from build123d import *

# Parameters (mm, degrees)
F0_W     = 152.4
F0_H     = 127
F1_DEPTH = 127
F2_W     = 101.6
F2_H     = 76.2
F3_DEPTH = 75.946
F4_R     = 23.2368410965
F5_DEPTH = 177.8
F6_R     = 38.1
F7_SIZE  = 35.56
F8_W     = 44.2467968255
F8_H     = 50.8
F9_DEPTH = 57.912


# Not quite as in the source:
# - a feature names something its author has since deleted; it is built from what else it names


with BuildPart() as f1:
    # F0 (on Front) → F1 (new body)
    with BuildSketch(Plane.XZ):
        Rectangle(F0_W, F0_H)
    extrude(amount=F1_DEPTH)

    # F2 (on face) → F3 (cut)
    with BuildSketch(Plane.XY.offset(63.5)):
        with Locations((25.4, -88.9)):
            Rectangle(F2_W, F2_H)
    extrude(amount=-F3_DEPTH, mode=Mode.SUBTRACT)

    # F4 (on face) → F5 (cut)
    with BuildSketch(Plane.XY.offset(-12.446)):
        with Locations((25.4, -88.9)):
            Circle(F4_R)
    extrude(amount=-F5_DEPTH, mode=Mode.SUBTRACT)

    # F6
    f6_edges = [f1.edges().sort_by_distance(p)[0] for p in [
        (-50.8, -127, 63.5),
    ]]
    fillet(f6_edges, radius=F6_R)

    # F7
    f7_edges = [f1.edges().sort_by_distance(p)[0] for p in [
        (76.2, -25.4, 63.5),
    ]]
    chamfer(f7_edges, length=F7_SIZE)

    # F8 (on face) → F9 (cut)
    with BuildSketch(Plane.XY.offset(63.5)):
        with Locations((-3.2766015872, -25.4)):
            Rectangle(F8_W, F8_H)
    extrude(amount=-F9_DEPTH, mode=Mode.SUBTRACT)


solid = f1.part
Design review of the part built by this model. Coordinates are the model's own, in mm. A direction names the side the tool comes from. Give positions to 0.01 mm unless a question says otherwise; leave off trailing zeros. Order: outer loops, then holes, each group sorted by start corner. A loop starts at its lowest first (then second) coordinate and runs counter-clockwise, first axis right, second up.
1. Add section A-A, the plane x = 25.4. State the section outline as (y, z) points.
Solution:
outline: (-127, -63.5) - (-112.14, -63.5) - (-112.14, -12.45) - (-127, -12.45) - close; (-65.66, -63.5) - (0, -63.5) - (0, 63.5) - (-50.8, 63.5) - (-50.8, -12.45) - (-65.66, -12.45) - close
2. Mouldability with a two-part tool opening along X and no side actions: class faces 1 (the flat face through (18.847, -26, 35)), 2 (the flat face through (58.67, -25.04, 45.47)), 3 (the flat face through (-51, -44, 63.5)) as +X half, -X half, draft (parallel to the pull), parting line (faces both ways), or undercut.
Solution:
face 1: undercut
face 2: +X half
face 3: draft
3. Add section B-B, the plane y = -30.5. State the section outline as (x, z) points.
Solution:
outline: (-76.2, -63.5) - (76.2, -63.5) - (76.2, 27.94) - (40.64, 63.5) - (18.85, 63.5) - (18.85, 5.59) - (-25.4, 5.59) - (-25.4, 63.5) - (-76.2, 63.5) - close
4. Add section C-C, the plane z = -36.5. State the section outline as (x, y) points.
Solution:
outline: (-76.2, -127) - (76.2, -127) - (76.2, 0) - (-76.2, 0) - close; hole circle Ø46.47 at (25.4, -88.9)
5. Add section D-D, the plane y = -97.5. State the section outline as (x, z) points, then the cut area to 3 significant figures.
Solution:
outline: (-76.2, -63.5) - (3.81, -63.5) - (3.81, -12.45) - (-25.4, -12.45) - (-25.4, 62.52) - (-76.2, 62.52) - close; (46.99, -63.5) - (76.2, -63.5) - (76.2, -12.45) - (46.99, -12.45) - close
area: 9,380 mm2
6. For pin 1 Ø5 at (x, y) = (58.5, -61) entering from +Z; pin 2 Ø6 at (x, z) = (20.5, -0.5) entering from +Y; pin 3 Ø5 at (y, z) = (-83, 49) entering from +X, all flat-tipped, find the tip position at first contact; note any pin that passes through.
Solution:
pin 1: stops at z = -12.45
pin 2: stops at y = 0
pin 3: stops at x = -25.4
7. To check wall thickness, follow L1, parallel to X at y = -47, z = 10; L2, parallel to X at y = -88, z = -49; L3, parallel to Y at x = 25.4, z = -29.5. State the ranges of each line that lie inside material, in increasing order.
Solution:
L1: x = -76.2 to -25.4, 18.85 to 76.2
L2: x = -76.2 to 2.18, 48.62 to 76.2
L3: y = -127 to -112.14, -65.66 to 0
8. Tool access review of faces 4 (the flat face through (30, -25, 63.5)), 5 (the flat face through (-4, -25, 5.588)), 6 (the flat face through (36, -50.8, 18)), 7 (the flat face through (-25.4, -64, 26)), 8 (the flat face through (-1, 0, -13)): name each direction out of +Z, -Z, +X, -X, +Y, -Y from which nothing blocks a thin tool from reaching the whole face with its end or side.
Solution:
face 4: +Z, +X, -X, +Y, -Y
face 5: +Z, +Y, -Y
face 6: +Z, +X, -Y
face 7: +Z, -Y
face 8: +Z, -Z, +X, -X, +Y
